from build123d import *

# Parameters (mm, degrees)
EXTRUDE_1_DEPTH = 5


with BuildPart() as part:
    # 草图1 → 凸台-拉伸1 (new body)
    with BuildSketch(Plane(origin=(0, 0, 0), x_dir=(1, 0, 0), z_dir=(0, 1, 0))):
        Polygon((0, 6), (0, 3), (2.544321256, 3), (2.544321256, 3.3), (22.544321256, 3.3), (22.544321256, 3), (40, 3), (40, 6), align=None)
        Polygon((2.544321256, 3), (0, 3), (0, 0), (40, 0), (40, 3), (22.544321256, 3), (22.544321256, 2.7), (2.544321256, 2.7), align=None)
    extrude(amount=EXTRUDE_1_DEPTH)


solid = part.part
Part model, mm, in its own coordinate system. A direction names the side the tool comes from. Coordinates: 2 decimals unless noted, no trailing zeros. Order: outer loops, then holes, each group sorted by start corner. A loop starts at its lowest first (then second) coordinate and runs counter-clockwise, first axis right, second up. Notation, with made-up numbers: M -18,-7 L -11,-7 A21 ccw -11,21 Z; hole C 88,80 d8. An arc over 180 degrees is marked long. Use a Markdown table: item, result.
(1) Probe L1, parallel to Z at x = 11, y = 4; L2, parallel to X at y = 4.7, z = -3.25. List the from-to ranges inside material, lowest first.
A:
| item | result |
|---|---|
| L1 | z = -6 to -3.3, -2.7 to 0 |
| L2 | x = 0 to 2.54, 22.54 to 40 |
(2) Pull direction X, two halves, no side cores. Call faces 3 (the flat face through (13, 2, -2.7)), 4 (the flat face through (20, 5, -4)), 5 (the flat face through (40, 2, -3)): released by +X, released by -X, zero draft, split by the parting line, or undercut.
A:
| item | result |
|---|---|
| face 3 | undercut |
| face 4 | zero draft |
| face 5 | released by +X |
(3) Cut at A-A on x = 6.5. Write the cut outline in (y, z).
A:
| item | result |
|---|---|
| outline | M 0,-6 L 5,-6 L 5,-3.3 L 0,-3.3 Z; M 0,-2.7 L 5,-2.7 L 5,0 L 0,0 Z |
(4) Cut at B-B on y = 1.1. Write the cut outline in (x, z).
A:
| item | result |
|---|---|
| outline | M 0,-6 L 40,-6 L 40,0 L 0,0 Z; hole M 2.54,-3.3 L 22.54,-3.3 L 22.54,-2.7 L 2.54,-2.7 Z |
(5) Tool access for faces 1 (the flat face through (12, 2, -3.3)), 2 (the flat face through (0, 2, -3)): list every direction of +Z, -Z, +X, -X, +Y, -Y with a clear straight run to the whole face (end or side of a thin tool).
A:
| item | result |
|---|---|
| face 1 | +Y, -Y |
| face 2 | +Z, -Z, -X, +Y, -Y |
